from build123d import *

# Parameters (mm, degrees)
SKETCH1_W           = 300
SKETCH1_H           = 100
BOSS_EXTRUDE1_DEPTH = 5
SKETCH7_R           = 10
BOSS_EXTRUDE5_DEPTH = 25
SKETCH10_R          = 4.5
CUT_EXTRUDE1_DEPTH  = 25


with BuildPart() as part:
    # Sketch1 → Boss-Extrude1 (new body)
    with BuildSketch(Plane(origin=(0, 0, 0), x_dir=(1, 0, 0), z_dir=(0, 1, 0))):
        Rectangle(SKETCH1_W, SKETCH1_H)
    extrude(amount=BOSS_EXTRUDE1_DEPTH)

    # Sketch7 → Boss-Extrude5 (add)
    with BuildSketch(Plane(origin=(150, 0, 0), x_dir=(0, 0, -1), z_dir=(1, 0, 0))):
        with Locations((50.954154719, 10.172311349)):
            Circle(SKETCH7_R)
    extrude(amount=-BOSS_EXTRUDE5_DEPTH)

    # Sketch10 → Cut-Extrude1 (cut)
    with BuildSketch(Plane(origin=(150, 0, 0), x_dir=(0, 0, -1), z_dir=(1, 0, 0))):
        with Locations((50.954154719, 10.172311349)):
            Circle(SKETCH10_R)
    extrude(amount=-CUT_EXTRUDE1_DEPTH, mode=Mode.SUBTRACT)


solid = part.part
For this review, take the finished solid that the model builds, in its own axes (mm). Coordinates: 2 decimals unless noted, no trailing zeros. Loops run counter-clockwise (first coordinate to the right, second up) from the corner with the lowest first, then second, coordinate; pieces in that order, holes last. Notation, with made-up numbers: (79, 2) - (88, 2) arc R20 ccw to (88, 38) - close; hole circle Ø9 at (50, -29). An arc over 180 degrees is marked (long way). Return JSON: item names as keys, results as strings.
Item 1: Take a section at A-A (z = -25). Give the boundary of the cut face in (x, y), then the cut area to 3 significant figures.
Determined:
{"outline": "(-150, 0) - (150, 0) - (150, 5) - (-150, 5) - close", "area": "1,500 mm2"}
Item 2: Insertion check: pin 1 (10 mm diameter, centred on x = -117, y = 5, fed in from -Z); pin 2 (6 mm diameter, centred on y = 8.5, z = -49.5, fed in from -X). Each pin has a flat end and moves straight along its axis. Give the tip position at first contact, or say it passes through.
Determined:
{"pin 1": "stops at z = -50", "pin 2": "stops at x = 125"}
Item 3: Mouldability with a two-part tool opening along Z and no side actions: class faces 1 (the flat face through (-2, 0, -1)), 2 (the flat face through (-2, 2, 50)), 3 (the cylindrical face through (137.68, 8.45, -55.11)) as pulls with the +Z half, pulls with the -Z half, needs draft (parallel to the pull), parting line crosses it, or undercut.
Determined:
{"face 1": "needs draft", "face 2": "pulls with the +Z half", "face 3": "undercut"}
Item 4: For line 1 (Y direction, x = -6, z = -25.5); line 2 (Z direction, x = 76.5, y = 3); line 3 (X direction, y = 15.25, z = -42.5), list the stretches that pass through material, from the lowest coordinate up.
Determined:
{"line 1": "y = 0 to 5", "line 2": "z = -50 to 50", "line 3": "x = 125 to 150"}
Item 5: Take a section at B-B (x = 52.5). Give the boundary of the cut face in (y, z), then the cut area to 3 significant figures.
Determined:
{"outline": "(0, -50) - (5, -50) - (5, 50) - (0, 50) - close", "area": "500 mm2"}
